Work out the finished part from the listing and answer in its coordinate system (mm). Face numbers are marked on the shaded views. A direction names the side the tool comes from. Round coordinates to 2 decimals unless told otherwise and drop trailing zeros. Write each loop counter-clockwise with the first axis right and the second up, starting at its lowest first coordinate (ties: lowest second). Pieces come first, ordered by that corner, then holes. Notation, with made-up numbers: M -1,21.25 L 20,21.25 A18 ccw 20,27.25 Z; hole C 54.5,78 d10. An arc over 180 degrees is marked long. One line per item, written item: value. Start each with the question number.
Q1. Consider probe 1 along Z at (x, y) = (19, 3.5); probe 2 along Y at (x, z) = (3.9, 56.05); probe 3 along Z at (x, y) = (20.75, 0). Determine where each line is inside the solid, lowest interval first.
Q2. Given pin 1 Ø2.5 at (x, y) = (21.5, -0.5) entering from +Z; pin 2 Ø1.8 at (x, y) = (20.9, 0) entering from +Z; pin 3 Ø1.5 at (y, z) = (1, 51.5) entering from +X; pin 4 Ø5 at (x, z) = (3, 63.5) entering from -Y, each flat-ended and moving along its own axis, determine where each tip first touches the part or whether it passes through.
Q3. Find section C-C (z = 24.5). Write down the section's boundary in (x, y), and give its area (3 significant figures).
Q4. Find section A-A (x = 3.75). Write down the section's boundary in (y, z), and give its area (3 significant figures).
Q5. Find section B-B (y = 0). Write down the section's boundary in (x, z), and give its area (3 significant figures).
Q6. Find section D-D (x = 13). Write down the section's boundary in (y, z).
Q7. A tool of negligible diameter and unlimited length cuts with its end or side. For the marked faces 1 and 2, from which of +Z, -Z, +X, -X, +Y, -Y can it reach the whole face along a straight path? Write none if from no direction.
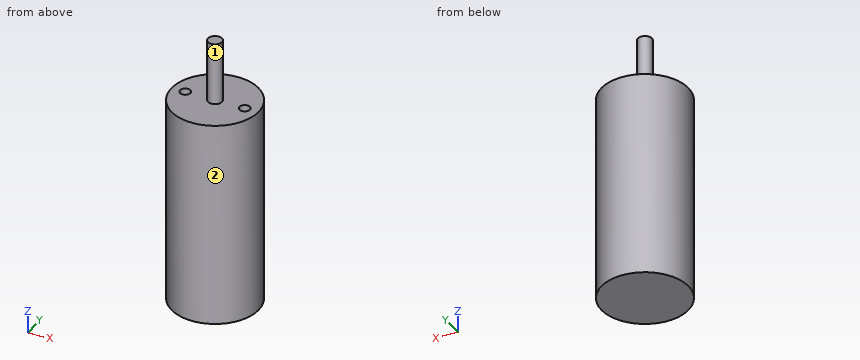
from build123d import *

# Parameters (mm, degrees)
SKETCH1_R           = 12.4
BOSS_EXTRUDE1_DEPTH = 59
SKETCH2_R           = 2
BOSS_EXTRUDE2_DEPTH = 17.8
SKETCH3_R           = 1.5
CUT_EXTRUDE1_DEPTH  = 4.3942


with BuildPart() as part:
    # Sketch1 → Boss-Extrude1 (new body)
    with BuildSketch(Plane.XY):
        with Locations((12.4, 0)):
            Circle(SKETCH1_R)
    extrude(amount=BOSS_EXTRUDE1_DEPTH)

    # Sketch2 → Boss-Extrude2 (add)
    with BuildSketch(Plane.XY.offset(59)):
        with Locations((12.4, 0)):
            Circle(SKETCH2_R)
    extrude(amount=BOSS_EXTRUDE2_DEPTH)

    # Sketch3 → Cut-Extrude1 (cut)
    with BuildSketch(Plane.XY.offset(59)):
        with Locations((20.9, 0)):
            Circle(SKETCH3_R)
        with Locations((3.9, 0)):
            Circle(SKETCH3_R)
    extrude(amount=-CUT_EXTRUDE1_DEPTH, mode=Mode.SUBTRACT)


solid = part.part
The answers:
1. probe 1: 0 to 59
1. probe 2: -9.03 to -1.5, 1.5 to 9.03
1. probe 3: 0 to 54.61
2. pin 1: z = 59
2. pin 2: z = 54.61
2. pin 3: x = 24.8
2. pin 4: through
3. outline: C 12.4,0 d24.8
3. area: 483 mm2
4. outline: M -8.88,0 L 8.88,0 L 8.88,59 L 1.49,59 L 1.49,54.61 L -1.49,54.61 L -1.49,59 L -8.88,59 Z
4. area: 1,040 mm2
5. outline: M 0,0 L 24.8,0 L 24.8,59 L 22.4,59 L 22.4,54.61 L 19.4,54.61 L 19.4,59 L 14.4,59 L 14.4,76.8 L 10.4,76.8 L 10.4,59 L 5.4,59 L 5.4,54.61 L 2.4,54.61 L 2.4,59 L 0,59 Z
5. area: 1,510 mm2
6. outline: M -12.39,0 L 12.39,0 L 12.39,59 L 1.91,59 L 1.91,76.8 L -1.91,76.8 L -1.91,59 L -12.39,59 Z
7. face 1: +Z
7. face 2: +Z, -Z
